Could you check a few things on this model? Use its own coordinates, in mm. Face numbers are marked on the shaded views. A direction names the side the tool comes from. Coordinates: 2 decimals unless noted, no trailing zeros. Loops run counter-clockwise (first coordinate to the right, second up) from the corner with the lowest first, then second, coordinate; pieces in that order, holes last. Notation, with made-up numbers: (54.5, 69) - (87.5, 69) arc R10 ccw to (87.5, 82) - close; hole circle Ø11 at (10.25, 4.25). An arc over 180 degrees is marked (long way). One line per item, written item: value. Start each with the question number.
(1) On a 3-axis mill with a long thin cutter (end or side, diameter ignored), from which of +Z, -Z, +X, -X, +Y, -Y can I reach the whole of each face in a straight line? I mean the marked faces 1, 2 and 3. Say none if no direction works.
(2) I'm going to push flat-ended pins straight in: P1, Ø10, axis at x = -40, z = 22.5, coming from the -Y side; P2, Ø8, axis at y = -4.5, z = 3, coming from the -X side; P3, Ø3, axis at x = 7.5, y = -9, coming from the +Z side; P4, Ø3, axis at x = -48.6, z = 27.01, coming from the +Y side. Where does each tip first touch, or does it pass through?
(3) If we section it at C-C on x = -48: Write out the boundary of the cut face in (y, z), then the cut area to 3 significant figures.
(4) If we section it at B-B on y = -7.75: Count the separate pieces of the cut face and the enclosed holes in it, then the cut area to 3 significant figures.
(5) If we mould it in two halves opening along Z, with no side actions, what happens to the marked faces 4, 5, 6 and 7? For each: pulls with the +Z half, pulls with the -Z half, needs draft (parallel to the pull), parting line crosses it, or undercut.
(6) If I drill on line 1 along Y through (x, z) = (-36.5, 21); line 2 along X through (y, z) = (-15.25, 12); line 3 along X through (y, z) = (-11.25, 23), over which ranges is the centre line in solid material (lowest first)? Write a range as from..to.
(7) If we section it at D-D on y = -18: Write out the boundary of the cut face in (x, z) (3 decimals).
(8) If we section it at A-A on z = 32: Write out the boundary of the cut face in (x, y), then the cut area to 3 significant figures.
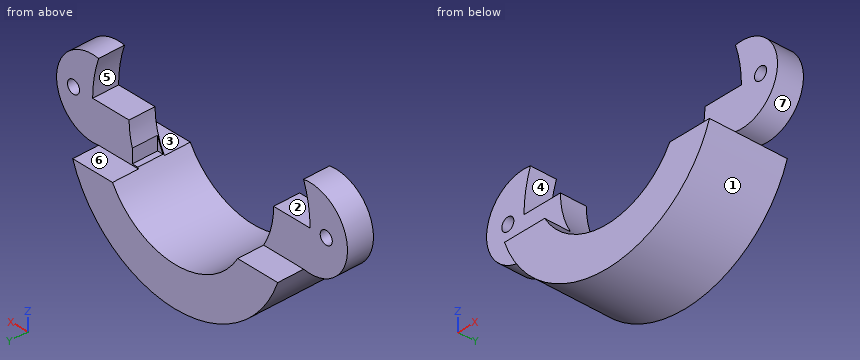
```python
from build123d import *

# Parameters (mm, degrees)
F0_R     = 1.5875
F1_DEPTH = 19.05
F2_R     = 1.5875
F3_DEPTH = 6.35
F4_R     = 1.5875
F5_DEPTH = 6.35
F8_DEPTH = 151.92272


with BuildPart() as f1:
    # F0 (on Front) → F1 (new body)
    with BuildSketch(Plane.XZ):
        with BuildLine():
            ThreePointArc((3.2306237647, 27.0146857947), (-15.7693382353, 8.0147237947), (-34.7693002353, 27.0146857947))
            Line((-34.7693002353, 27.0146857947), (-44.3443382353, 27.0146857947))
            ThreePointArc((-44.3443382353, 27.0146857947), (-43.9176321109, 31.9344598635), (-42.6502576132, 36.7073014581))
            ThreePointArc((-42.6502576132, 36.7073014581), (-54.1838863729, 27.0146857947), (-42.6502576132, 17.3220701313))
            ThreePointArc((-42.6502576132, 17.3220701313), (-15.5884947503, -1.5597419447), (11.2321092838, 17.6630839601))
            ThreePointArc((11.2321092838, 17.6630839601), (22.288726896, 27.0146857947), (11.2321092838, 36.3662876293))
            ThreePointArc((11.2321092838, 36.3662876293), (12.4095278514, 31.7562183603), (12.8056617647, 27.0146857947))
            Line((12.8056617647, 27.0146857947), (3.2306237647, 27.0146857947))
        make_face()
        with Locations((-48.6005805433, 27.0146857947)):
            Circle(F0_R, mode=Mode.SUBTRACT)
        with Locations((17.8374499083, 27.0146857947)):
            Circle(F0_R, mode=Mode.SUBTRACT)
    extrude(amount=F1_DEPTH)

    # F2 (on face) → F3 (cut)
    with BuildSketch(Plane.XZ.offset(19.05)):
        with BuildLine():
            ThreePointArc((-42.6502576132, 36.7073014581), (-54.1838863729, 27.0146857947), (-42.6502576132, 17.3220701313))
            Line((-42.6502576132, 17.3220701313), (-32.1110565538, 17.3220701313))
            ThreePointArc((-32.1110565538, 17.3220701313), (-34.0926919549, 21.989423168), (-34.7693002353, 27.0146857947))
            Line((-34.7693002353, 27.0146857947), (-44.3443382353, 27.0146857947))
            ThreePointArc((-44.3443382353, 27.0146857947), (-43.9176321109, 31.9344598635), (-42.6502576132, 36.7073014581))
        make_face()
        with Locations((-48.6005805433, 27.0146857947)):
            Circle(F2_R, mode=Mode.SUBTRACT)
        with BuildLine():
            Line((0.7698908619, 17.6630839601), (11.2321092838, 17.6630839601))
            ThreePointArc((11.2321092838, 17.6630839601), (22.288726896, 27.0146857947), (11.2321092838, 36.3662876293))
            ThreePointArc((11.2321092838, 36.3662876293), (12.4095278514, 31.7562183603), (12.8056617647, 27.0146857947))
            Line((12.8056617647, 27.0146857947), (3.2306237647, 27.0146857947))
            ThreePointArc((3.2306237647, 27.0146857947), (2.6051451637, 22.1797177676), (0.7698908619, 17.6630839601))
        make_face()
        with Locations((17.8374499083, 27.0146857947)):
            Circle(F2_R, mode=Mode.SUBTRACT)
    extrude(amount=-F3_DEPTH, mode=Mode.SUBTRACT)

    # F4 (on face) → F5 (cut)
    with BuildSketch(Plane(origin=(0, 0, 0), x_dir=(-1, 0, 0), z_dir=(0, 1, 0))):
        with BuildLine():
            ThreePointArc((-11.2321092838, 36.3662876293), (-22.288726896, 27.0146857947), (-11.2321092838, 17.6630839601))
            Line((-11.2321092838, 17.6630839601), (-0.7698908619, 17.6630839601))
            ThreePointArc((-0.7698908619, 17.6630839601), (-2.6051451637, 22.1797177676), (-3.2306237647, 27.0146857947))
            Line((-3.2306237647, 27.0146857947), (-12.8056617647, 27.0146857947))
            ThreePointArc((-12.8056617647, 27.0146857947), (-12.4095278514, 31.7562183603), (-11.2321092838, 36.3662876293))
        make_face()
        with Locations((-17.8374499083, 27.0146857947)):
            Circle(F4_R, mode=Mode.SUBTRACT)
        with BuildLine():
            Line((32.134551767, 17.3617928572), (42.6502576132, 17.3220701313))
            ThreePointArc((42.6502576132, 17.3220701313), (54.1838863729, 27.0146857947), (42.6502576132, 36.7073014581))
            ThreePointArc((42.6502576132, 36.7073014581), (43.9176321109, 31.9344598635), (44.3443382353, 27.0146857947))
            Line((44.3443382353, 27.0146857947), (34.7693002353, 27.0146857947))
            ThreePointArc((34.7693002353, 27.0146857947), (34.0987816423, 22.011680659), (32.134551767, 17.3617928572))
        make_face()
        with Locations((48.6005805433, 27.0146857947)):
            Circle(F4_R, mode=Mode.SUBTRACT)
    extrude(amount=-F5_DEPTH, mode=Mode.SUBTRACT)

    # F7 (on offset) → F8 (cut)
    with BuildSketch(Plane(origin=(-0.6417229615, 0, 169.8818432743), x_dir=(0.9999928655, 0, 0.0037774395), z_dir=(-0.0037774395, 0, 0.9999928655))):
        Polygon((2.4513369426, -5.8165588416), (-31.672719866, -5.8165588416), (-31.3653349876, -12.5274714082), (2.4513369426, -12.5274714082), align=None)
    extrude(amount=-F8_DEPTH, mode=Mode.SUBTRACT)


solid = f1.part
```
Values:
1. face 1: -Z, +Y, -Y
1. face 2: +Y, -Y
1. face 3: +Z, +X, -X, -Y
2. P1: stops at y = -12.7
2. P2: stops at x = -36.16
2. P3: stops at z = 27.01
2. P4: passes through
3. outline: (-12.7, 17.88) - (-6.35, 17.88) - (-6.35, 25.55) - (-12.7, 25.55) - close; (-12.7, 28.48) - (-6.35, 28.48) - (-6.35, 36.15) - (-12.7, 36.15) - close
3. area: 97.4 mm2
4. separate pieces: 1
4. enclosed holes: 2
4. area: 1,010 mm2
5. face 4: undercut
5. face 5: undercut
5. face 6: pulls with the +Z half
5. face 7: parting line crosses it
6. line 1: y = -12.7..-6.35
6. line 2: x = -40.08..-27.41, -4.13..8.54
6. line 3: x = -53.33..-34.34, 2.8..21.4
7. outline: (-42.65, 17.322) arc R28.575 ccw to (11.232, 17.663) - (0.77, 17.663) arc R19 cw to (-32.111, 17.322) - close
8. outline: (-52.83, -12.7) - (-43.91, -12.7) - (-43.91, -6.35) - (-52.83, -6.35) - close; (12.37, -12.7) - (20.87, -12.7) - (20.87, -6.35) - (12.37, -6.35) - close
8. area: 111 mm2
